Could you check a few things on this model? Use its own coordinates, in mm. A direction names the side the tool comes from. Coordinates: 2 decimals unless noted, no trailing zeros. Loops run counter-clockwise (first coordinate to the right, second up) from the corner with the lowest first, then second, coordinate; pieces in that order, holes last.
1) Will these pins go through, and if not, where does the flat tip stop? P1, Ø1.3, axis at x = 11.5, y = -24, coming from the +Z side; P2, Ø3, axis at y = -25, z = 2.5, coming from the +X side; P3, Ø0.8, axis at y = -24.5, z = 2, coming from the -X side.
2) If I drill on line 1 along X through (y, z) = (-9, 9.5); line 2 along X through (y, z) = (0, 3.25); line 3 along Z through (x, y) = (-1.27, -20.75) (3 decimals), over which ranges is the centre line in solid material (lowest first)?
3) Thinking about a two-plate mould opening in X: for faces 1 (the face through (-0.01, -18.44, 2.07)), 2 (the face through (13.208, -24, 2)), 3 (the face through (11, -24, 3.683)), 4 (the face through (9.652, -24, 2)), which applies, released by +X, released by -X, zero draft, split by the parting line, or undercut?
4) Imagine slicing it at C-C on x = -1.27. Please give me the cut outline in (y, z) (3 decimals).
5) Imagine slicing it at A-A on z = 1.5. Please give me the cut outline in (x, y), plus the area to 3 significant figures.
6) Imagine slicing it at D-D on z = 6. Please give me the cut outline in (x, y).
7) Imagine slicing it at B-B on y = -3. Please give me the cut outline in (x, z).
8) For faces 5 (the face through (-14, -24, 3.683)), 6 (the face through (-14, -24, 0.127)), 7 (the face through (-15.748, -24, 2)), which set-ups out of +Z, -Z, +X, -X, +Y, -Y let a thin tool reach every point of the face, with its end or its side?
```python
from build123d import *

# Parameters (mm, degrees)
BOSS_EXTRUDE1_DEPTH = 12.7
SKETCH2_W           = 3.556
SKETCH2_H           = 3.556
BOSS_EXTRUDE2_DEPTH = 2.54
SKETCH3_R           = 1.27
CUT_EXTRUDE1_DEPTH  = 14.986


with BuildPart() as part:
    # Sketch1 → Boss-Extrude1 (new body)
    with BuildSketch(Plane.XY):
        with BuildLine():
            Line((-38.1, 23.241), (-38.1, -23.241))
            Line((-38.1, -23.241), (38.1, -23.241))
            Line((38.1, -23.241), (38.1, 23.241))
            Line((38.1, 23.241), (36.83, 23.241))
            ThreePointArc((36.83, 23.241), (0, -13.589), (-36.83, 23.241))
            Line((-36.83, 23.241), (-38.1, 23.241))
        make_face()
    extrude(amount=BOSS_EXTRUDE1_DEPTH)

    # Sketch2 → Boss-Extrude2 (add)
    with BuildSketch(Plane.XZ.offset(23.241)):
        with Locations((11.43, 1.905)):
            Rectangle(SKETCH2_W, SKETCH2_H)
        with Locations((-13.97, 1.905)):
            Rectangle(SKETCH2_W, SKETCH2_H)
    extrude(amount=BOSS_EXTRUDE2_DEPTH)

    # Sketch3 → Cut-Extrude1 (cut)
    with BuildSketch(Plane(origin=(0, -23.241, 0), x_dir=(-1, 0, 0), z_dir=(0, -1, 0))):
        with Locations(Location((1.27, -1.905, 0), (0, 0, 90))):
            Circle(SKETCH3_R)
    extrude(amount=-CUT_EXTRUDE1_DEPTH, mode=Mode.SUBTRACT)


solid = part.part
```
Filled in:
1. P1: stops at z = 3.68
1. P2: stops at x = 13.21
1. P3: stops at x = -15.75
2. line 1: x = -38.1 to -17.8, 17.8 to 38.1
2. line 2: x = -38.1 to -28.57, 28.57 to 38.1
2. line 3: z = 0 to 0.635, 3.175 to 12.7
3. face 1: undercut
3. face 2: released by +X
3. face 3: zero draft
3. face 4: undercut
4. outline: (-23.241, 0) - (-13.567, 0) - (-13.567, 0.635) - (-23.241, 0.635) - close; (-23.241, 3.175) - (-13.567, 3.175) - (-13.567, 12.7) - (-23.241, 12.7) - close
5. outline: (-38.1, -23.24) - (-15.75, -23.24) - (-15.75, -25.78) - (-12.19, -25.78) - (-12.19, -23.24) - (-2.47, -23.24) - (-2.47, -13.51) arc R36.83 cw to (-36.83, 23.24) - (-38.1, 23.24) - close; (-0.07, -23.24) - (9.65, -23.24) - (9.65, -25.78) - (13.21, -25.78) - (13.21, -23.24) - (38.1, -23.24) - (38.1, 23.24) - (36.83, 23.24) arc R36.83 cw to (-0.07, -13.59) - close
5. area: 1,410 mm2
6. outline: (-38.1, -23.24) - (38.1, -23.24) - (38.1, 23.24) - (36.83, 23.24) arc R36.83 cw to (-36.83, 23.24) - (-38.1, 23.24) - close
7. outline: (-38.1, 0) - (-25.84, 0) - (-25.84, 12.7) - (-38.1, 12.7) - close; (25.84, 0) - (38.1, 0) - (38.1, 12.7) - (25.84, 12.7) - close
8. face 5: +Z, +X, -X, -Y
8. face 6: -Z, +X, -X, -Y
8. face 7: +Z, -Z, -X, -Y
